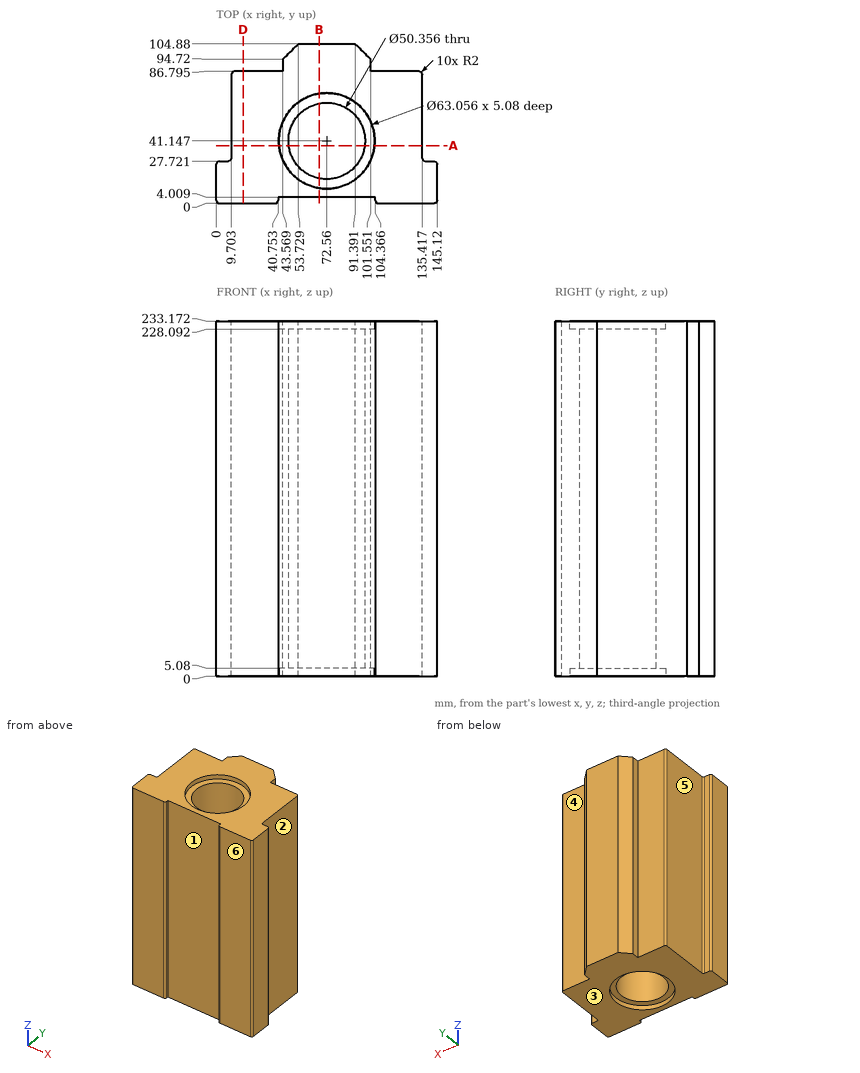
Here's the drawing with two shaded views (mm, measured from the low corner). I have some questions. A direction names the side the tool comes from. Coordinates: 2 decimals unless noted, no trailing zeros. Write each loop counter-clockwise with the first axis right and the second up, starting at its lowest first coordinate (ties: lowest second). Pieces come first, ordered by that corner, then holes. Notation, with made-up numbers: M 76.25,11.25 L 100.25,11.25 A34 cw 100.25,41.25 Z; hole C 76,68.25 d5. An arc over 180 degrees is marked long. Answer as CSV lines item,"result". Start each with the question number.
1) I want a section at B-B, the plane x = 67.5. Please give me the cut outline in (y, z).
2) Please list where these lines run through material, in increasing order: line 1 (Y direction, x = 71.5, z = 222); line 2 (X direction, y = 67, z = 17); line 3 (X direction, y = 42, z = 145.5). Write a range as from..to.
3) I want a section at A-A, the plane y = 38. Please give me the cut outline in (x, z), and give its area (3 significant figures).
4) I want a section at D-D, the plane x = 17.5. Please give me the cut outline in (y, z) (1 decimal).
5) We'd pull the mould along X, two halves only. Please class the marked faces 1, 2 and 3: +X half, -X half, draft (parallel to the pull), parting line (faces both ways), or undercut.
6) For P1, Ø9.5, axis at x = 115, z = 171.5, coming from the +Y side (1 decimal); P2, Ø2.5, axis at y = 89.5, z = 85, coming from the +X side; P3, Ø8, axis at y = 17.5, z = 113.5, coming from the -X side; P4, Ø4.5, axis at x = 5, z = 111, coming from the +Y side, each with a flat end and sliding along its axis, tell me the tip position at first contact or that it passes through.
7) For the marked faces 4, 5 and 6, which set-ups out of +Z, -Z, +X, -X, +Y, -Y let a thin tool reach every point of the face, with its end or its side?
Data:
1,outline,"M 4.01,0 L 10.03,0 L 10.03,5.08 L 16.48,5.08 L 16.48,228.09 L 10.03,228.09 L 10.03,233.17 L 4.01,233.17 Z; M 65.81,5.08 L 72.27,5.08 L 72.27,0 L 104.88,0 L 104.88,233.17 L 72.27,233.17 L 72.27,228.09 L 65.81,228.09 Z"
2,line 1,"y = 4.01..15.99, 66.3..104.88"
2,line 2,"x = 9.7..135.42"
2,line 3,"x = 9.7..47.4, 97.72..135.42"
3,outline,"M 9.7,0 L 41.19,0 L 41.19,5.08 L 47.58,5.08 L 47.58,228.09 L 41.19,228.09 L 41.19,233.17 L 9.7,233.17 Z; M 97.54,5.08 L 103.93,5.08 L 103.93,0 L 135.42,0 L 135.42,233.17 L 103.93,233.17 L 103.93,228.09 L 97.54,228.09 Z"
3,area,"17,500 mm^2"
4,outline,"M 0,0 L 86.8,0 L 86.8,233.2 L 0,233.2 Z"
5,face 1,"undercut"
5,face 2,"+X half"
5,face 3,"draft"
6,P1,"stops at y = 86.8"
6,P2,"stops at x = 101.55"
6,P3,"stops at x = 0"
6,P4,"stops at y = 27.72"
7,face 4,"+Z, -Z, +X, +Y"
7,face 5,"+Z, -Z, -X, +Y"
7,face 6,"+Z, -Z, +X, -X, -Y"
